from build123d import *

# Parameters (mm, degrees)
CROQUIS1_W              = 1
CROQUIS1_H              = 74
CROQUIS1_H_2            = 1
CROQUIS1_W_2            = 190
SALIENTE_EXTRUIR1_DEPTH = 20
SALIENTE_EXTRUIR2_DEPTH = 1
CORTAR_EXTRUIR1_DEPTH   = 225.75375414
CROQUIS4_W              = 71
CROQUIS4_H              = 20
SALIENTE_EXTRUIR3_DEPTH = 1


with BuildPart() as part:
    # Croquis1 → Saliente-Extruir1 (new body)
    with BuildSketch(Plane(origin=(0, 0, 0), x_dir=(1, 0, 0), z_dir=(0, 1, 0))):
        with Locations((-95.5, 37.5)):
            Rectangle(CROQUIS1_W, CROQUIS1_H)
        with Locations((-95.5, 0)):
            Rectangle(CROQUIS1_W, CROQUIS1_H_2)
        Rectangle(CROQUIS1_W_2, CROQUIS1_H_2)
        with Locations((95.5, 37.5)):
            Rectangle(CROQUIS1_W, CROQUIS1_H)
        with Locations((95.5, 0)):
            Rectangle(CROQUIS1_W, CROQUIS1_H_2)
    extrude(amount=SALIENTE_EXTRUIR1_DEPTH)

    # Croquis2 → Saliente-Extruir2 (add)
    with BuildSketch(Plane.ZY.offset(96)):
        Polygon((12.544924521, 90), (-61.219684248, 20), (-32.164890823, 20), (12.544924521, 62.428030546), align=None)
        Polygon((-61.219684248, 20), (-74.5, 7.397450917), (-67.480081196, 0), (-53.240493329, 0), (-32.164890823, 20), align=None)
    extrude(amount=-SALIENTE_EXTRUIR2_DEPTH)

    # Croquis3 → Cortar-Extruir1 (cut, through all)
    with BuildSketch(Plane.ZY.offset(96)):
        Polygon((-61.219684248, 20), (-74.5, 3.892353298), (-74.5, 20), align=None)
    extrude(amount=-CORTAR_EXTRUIR1_DEPTH, mode=Mode.SUBTRACT)

    # Croquis4 → Saliente-Extruir3 (add)
    with BuildSketch(Plane.ZY.offset(96)):
        with Locations((48.044924521, 80)):
            Rectangle(CROQUIS4_W, CROQUIS4_H)
    extrude(amount=-SALIENTE_EXTRUIR3_DEPTH)


solid = part.part
Verification items for the finished model (mm, model axes). A direction names the side the tool comes from. Coordinates: 2 decimals unless noted, no trailing zeros. Loops run counter-clockwise (first coordinate to the right, second up) from the corner with the lowest first, then second, coordinate; pieces in that order, holes last. Notation, with made-up numbers: M 14,24 L 71,24 A32 cw 71,53 Z; hole C -30.75,-20 d4. An arc over 180 degrees is marked long. One line per item, written item: value.
1. Set-up check for faces 1 (the flat face through (-95.507, 12.059, -67.767)), 2 (the flat face through (95, 10, -37)), 3 (the flat face through (-95.51, 40.92, -10.12)): record each of +Z, -Z, +X, -X, +Y, -Y from which the full face is reachable in a straight line by a thin tool's end or side.
Answers follow:
face 1: -Z, +X, -X, +Y
face 2: -Z, +Y, -Y
face 3: +Z, +X, -X
2. Mould release check, pull along X, two halves, no side actions. Record for faces 4 (the flat face through (95.493, 12.059, -67.767)), 5 (the flat face through (-1, 10, -0.5)), 6 (the flat face through (-96, 52, -8)): pulls with the +X half, pulls with the -X half, needs draft (parallel to the pull), parting line crosses it, or undercut.
Answers follow:
face 4: needs draft
face 5: undercut
face 6: pulls with the -X half
3. Section check C-C on z = -28. Record the cut outline in (x, y), plus the area to 3 significant figures.
Answers follow:
outline: M -96,0 L -95,0 L -95,20 L -96,20 Z; M -96,23.95 L -95,23.95 L -95,51.52 L -96,51.52 Z; M 95,0 L 96,0 L 96,20 L 95,20 Z
area: 67.6 mm^2
4. Gauge pin test, flat ends, axial feed: P1, Ø2, axis at y = 28.5, z = -50, coming from the +X side; P2, Ø10, axis at x = -45, y = 15, coming from the +Z side; P3, Ø22, axis at x = 27.5, y = 5, coming from the -Z side. Record the tip position at first contact, or that the pin passes through.
Answers follow:
P1: x = -95
P2: z = 0.5
P3: z = -0.5
5. Material ranges on line 1 along X through (y, z) = (5, -29.5); line 2 along X through (y, z) = (37, -24), recorded low to high. Write a range as from..to.
Answers follow:
line 1: -96..-95, 95..96
line 2: -96..-95
6. Section check A-A on z = -48. Record the cut outline in (x, y).
Answers follow:
outline: M -96,0 L -95,0 L -95,32.55 L -96,32.55 Z; M 95,0 L 96,0 L 96,20 L 95,20 Z
7. Section check D-D on x = -16.5. Record the cut outline in (y, z), plus the area to 3 significant figures.
Answers follow:
outline: M 0,-0.5 L 20,-0.5 L 20,0.5 L 0,0.5 Z
area: 20.0 mm^2
8. Section check B-B on y = 9. Record the cut outline in (x, z).
Answers follow:
outline: M -96,-70.29 L -95,-70.29 L -95,-0.5 L 95,-0.5 L 95,-70.29 L 96,-70.29 L 96,0.5 L -96,0.5 Z
